Autodesk Fusion 360 part; units mm, degrees
sketch "Plate" plane through (0, 0, 0) normal (0, 1, 0) x (1, 0, 0)
  circle A0 centre (0, 0) radius 21.5
  circle A1 centre (0, 0) radius 20
  line L0 (5, -23) -> (-5, -23)
  line L1 (-5, -23) -> (-5, 23)
  line L2 (-5, 23) -> (5, 23)
  line L3 (5, 23) -> (5, -23)
  line L4 (23, -5) -> (-23, -5)
  line L5 (-23, -5) -> (-23, 5)
  line L6 (-23, 5) -> (23, 5)
  line L7 (23, 5) -> (23, -5)
  line L8 (7.5, -7.5) -> (-7.5, -7.5) construction
  line L9 (-7.5, -7.5) -> (-7.5, 7.5) construction
  line L10 (-7.5, 7.5) -> (7.5, 7.5) construction
  line L11 (7.5, 7.5) -> (7.5, -7.5) construction
  line L12 (7.5, -7.5) -> (-7.5, 7.5) construction
  line L13 (-7.5, -7.5) -> (7.5, 7.5) construction
  circle A2 centre (7.5, 7.5) radius 1
  circle A3 centre (7.5, -7.5) radius 1
  circle A4 centre (-7.5, -7.5) radius 1
  circle A5 centre (-7.5, 7.5) radius 1
  circle A6 centre (2.5, -5) radius 0.9
  circle A7 centre (-8.5, 15.5) radius 0.9
  dimension "d1" = 43
  dimension "d2" = 40
  dimension "d3" = 10
  dimension "d4" = 46
  dimension "d5" = 10
  dimension "d6" = 15
  dimension "d7" = 15
  dimension "d8" = 2
  dimension "d9" = 2
  dimension "d10" = 2
  dimension "d11" = 2
  dimension "d12" = 1.8
  dimension "d13" = 1.8
extrude "Extrude1" add sketch "Plate" against normal blind 2 contours A0 A1 L4 L6 | A0 A1 L1 L3 | A1 L3 L6 | A1 L3 L4 L6 | A0 A1 L1 L3 | A1 L3 L4 | A1 L1 L3 L6 | L1 L3 L4 L6 A6 | A1 L1 L3 L4 A6 | A0 A1 L4 L6 | A1 L1 L6 | A1 L1 L4 L6 | A1 L1 L4
sketch "Buttons" plane through (0, 0, 0) normal (0, 1, 0) x (1, 0, 0)
  line L0 (16, -3.25) -> (12, -3.25)
  line L1 (12, -3.25) -> (12, 3.25)
  line L2 (12, 3.25) -> (16, 3.25)
  line L3 (16, 3.25) -> (16, -3.25)
  line L4 (16, -3.25) -> (12, 3.25) construction
  line L5 (12, -3.25) -> (16, 3.25) construction
  circle A0 centre (14, 3.25) radius 1
  circle A1 centre (14, -3.25) radius 1
  circle A2 centre (-3.25, 14) radius 1
  circle A3 centre (3.25, 14) radius 1
  line L6 (3.25, 12) -> (-3.25, 12)
  line L7 (-3.25, 12) -> (-3.25, 16)
  line L8 (3.25, 16) -> (3.25, 12)
  line L9 (-3.25, 16) -> (3.25, 16)
  circle A4 centre (-14, -3.25) radius 1
  circle A5 centre (-14, 3.25) radius 1
  line L10 (-12, 3.25) -> (-12, -3.25)
  line L11 (-12, -3.25) -> (-16, -3.25)
  line L12 (-16, 3.25) -> (-12, 3.25)
  line L13 (-16, -3.25) -> (-16, 3.25)
  circle A6 centre (3.25, -14) radius 1
  circle A7 centre (-3.25, -14) radius 1
  line L14 (-3.25, -12) -> (3.25, -12)
  line L15 (3.25, -12) -> (3.25, -16)
  line L16 (-3.25, -16) -> (-3.25, -12)
  line L17 (3.25, -16) -> (-3.25, -16)
  point P0 (14, 0)
  dimension "d16" = 4
  dimension "d17" = 6.5
  dimension "d18" = 2
  dimension "d19" = 2
  dimension "d21" = 360
extrude "Extrude2" cut sketch "Buttons" against normal blind 1.8 contours L0 L1 L2 L3 A0 A1 | A2 A3 L6 L7 L8 L9 | A4 A5 L10 L11 L12 L13 | A6 A7 L14 L15 L16 L17
extrude "Extrude3" cut sketch "Buttons" against normal blind 3 contours L0 A1 | L0 A1 | L2 A0 | L2 A0 | A2 L7 | A2 L7 | A3 L8 | A3 L8 | A4 L11 | A4 L11 | A5 L12 | A5 L12 | A6 L15 | A6 L15 | A7 L16 | A7 L16
Geometry check sheet. Reference: the model listing, model coordinates, mm. A direction names the side the tool comes from. Give positions to 0.01 mm unless a question says otherwise; leave off trailing zeros. Order: outer loops, then holes, each group sorted by start corner. A loop starts at its lowest first (then second) coordinate and runs counter-clockwise, first axis right, second up. Notation, with made-up numbers: (72.5, 83.25) - (120.5, 83.25) arc R26 ccw to (120.5, 119.25) - close; hole circle Ø8 at (-20, 64). An arc over 180 degrees is marked (long way). Answer as a JSON object with one key per item and string values.
(1) Draft check along Z on faces 4 (the cylindrical face through (-14.036, -0.986, -14.247)), 5 (the cylindrical face through (-7.63, -0.99, 6.51)), 6 (the flat face through (-5, -1, 20)), 7 (the cylindrical face through (-14.13, -0.99, -4.24)). Enter one of: released by +Z, released by -Z, zero draft, split by the parting line, or undercut.
Report:
{"face 4": "released by -Z", "face 5": "undercut", "face 6": "zero draft", "face 7": "undercut"}
(2) Cross-section at D-D (z = -5.5). Record the cut outline in (x, y), then the cut area to 3 significant figures.
Report:
{"outline": "(-19.23, -2) - (19.23, -2) - (19.23, 0) - (-19.23, 0) - close", "area": "76.9 mm^2"}
(3) Tool access check on faces 1 (the cylindrical face through (0.1, -1, -21.5)), 2 (the flat face through (-20, -1, -5)), 3 (the flat face through (12.5, -0.9, -3.25)). Record the directions out of +Z, -Z, +X, -X, +Y, -Y that give a thin tool (end or side, any length) a straight path to the whole face; none if there is none.
Report:
{"face 1": "-Z, +Y, -Y", "face 2": "-Z, -X, +Y, -Y", "face 3": "+Y"}
(4) Material ranges on line 1 (X direction, y = -1.05, z = -7.5); line 2 (Z direction, x = 7, y = -0.85) (3 decimals), recorded low to high.
Report:
{"line 1": "-18.54 to -8.5, -6.5 to 6.5, 8.5 to 18.54", "line 2": "-18.735 to -8.366, -6.634 to 6.634, 8.366 to 18.735"}
(5) Cross-section at B-B (x = 14). Record the cut outline in (y, z).
Report:
{"outline": "(-2, -14.28) - (0, -14.28) - (0, -4.25) - (-2, -4.25) - close; (-2, -2.25) - (-1.8, -2.25) - (-1.8, 2.25) - (-2, 2.25) - close; (-2, 4.25) - (0, 4.25) - (0, 14.28) - (-2, 14.28) - close"}
(6) Depth check by flat-ended pin: pin 1 Ø0.5 at (x, y) = (12.5, -0.5) entering from +Z; pin 2 Ø0.5 at (y, z) = (-0.5, 0.5) entering from -X; pin 3 Ø0.9 at (x, y) = (-1.5, -1) entering from -Z. Enter the tip coordinate at first touch or a pass-through.
Report:
{"pin 1": "z = 15.81", "pin 2": "x = -21.5", "pin 3": "z = -21.47"}
(7) Cross-section at A-A (z = 14.5). Record the cut outline in (x, y).
Report:
{"outline": "(-13.77, -2) - (-4.12, -2) - (-4.12, 0) - (-13.77, 0) - close; (-2.38, -2) - (2.38, -2) - (2.38, -1.8) - (-2.38, -1.8) - close; (4.12, -2) - (13.77, -2) - (13.77, 0) - (4.12, 0) - close"}
(8) Cross-section at C-C (y = -0.35). State how many separate pieces and enclosed holes the cut face has, then the cut area to 3 significant figures.
Report:
{"separate pieces": "1", "enclosed holes": "10", "area": "1,180 mm^2"}
